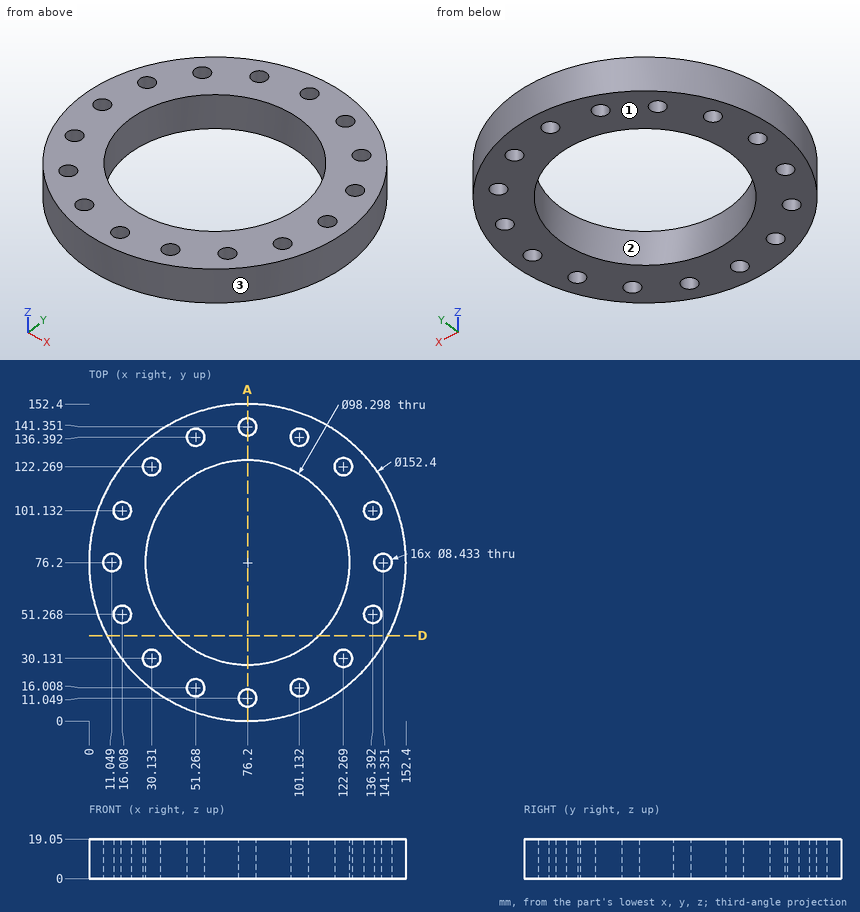
Design review of the part shown in the three views and the two pictorial views. Dimensions are in mm from the part's minimum x, y and z. Round coordinates to 2 decimals unless told otherwise and drop trailing zeros. Loops run counter-clockwise (first coordinate to the right, second up) from the corner with the lowest first, then second, coordinate; pieces in that order, holes last. Notation, with made-up numbers: (-30.75, 70.25) -> (4.25, 70.25) arc R19 ccw to (4.25, 81.25) -> close; hole circle Ø11 at (-33, 45). An arc over 180 degrees is marked (long way). Answer as a JSON object with one key per item and string values. Group by question number.
1) For pin 1 Ø7.5 at (x, y) = (122.27, 122.27) entering from +Z; pin 2 Ø6 at (x, z) = (122.5, 11) entering from +Y; pin 3 Ø8 at (x, z) = (33.5, 8) entering from -Y; pin 4 Ø1 at (x, z) = (121, 6.5) entering from +Y, all flat-tipped, find the tip position at first contact; note any pin that passes through.
2) For line 1 (Y direction, x = 26.5, z = 12) (1 decimal); line 2 (Y direction, x = 133.5, z = 4.5) (1 decimal); line 3 (X direction, y = 74, z = 17.25) (1 decimal), list the stretches that pass through material, from the lowest coordinate up. Write a range as [from, to].
3) Mouldability with a two-part tool opening along Y and no side actions: class the marked faces 1, 2 and 3 as released by +Y, released by -Y, zero draft, split by the parting line, or undercut.
4) We need section D-D on y = 41. Write out the cut boundary in (x, z), then the cut area to 3 significant figures.
5) We need section A-A on x = 76.2. Give the number of separate pieces and of enclosed holes in the cut face.
Result set:
{
 "1": {"pin 1": "through", "pin 2": "y = 138.9", "pin 3": "y = 10.56", "pin 4": "y = 138.2"},
 "2": {"line 1": "[18.4, 28], [32.3, 120.1], [124.4, 134]", "line 2": "[26, 48.2], [54.3, 98.1], [104.2, 126.4]", "line 3": "[0, 7.5], [14.6, 27.1], [125.3, 137.8], [144.9, 152.4]"},
 "3": {"face 1": "zero draft", "face 2": "undercut", "face 3": "split by the parting line"},
 "4": {"outline": "(8.62, 0) -> (41.9, 0) -> (41.9, 19.05) -> (8.62, 19.05) -> close; (110.5, 0) -> (143.78, 0) -> (143.78, 19.05) -> (110.5, 19.05) -> close", "area": "1,270 mm²"},
 "5": {"separate pieces": "4", "enclosed holes": "0"}
}
